Work out the finished part from the listing and answer in its coordinate system (mm). A direction names the side the tool comes from. Give positions to 0.01 mm unless a question says otherwise; leave off trailing zeros. Loops run counter-clockwise (first coordinate to the right, second up) from the corner with the lowest first, then second, coordinate; pieces in that order, holes last. Notation, with made-up numbers: M -36.75,63 L 13.25,63 A28 ccw 13.25,89 Z; hole C 53,-11 d11. An arc over 180 degrees is marked long. Write item = value, one per line. Start each with the question number.
1. Section B-B on x = 0 is taken. Determine the outline of the cut face in (y, z) (1 decimal).
2. Section D-D on y = -59 is taken. Determine the outline of the cut face in (x, z) (3 decimals).
3. Section C-C on y = -7 is taken. Determine the outline of the cut face in (x, z).
4. Flat-ended cylindrical pins translate along their axes: pin 1 Ø12 at (x, z) = (21, 14.5) entering from -Y; pin 2 Ø4 at (y, z) = (-84, 22) entering from +X; pin 3 Ø2 at (x, z) = (11, -22.5) entering from -Y; pin 4 Ø6 at (y, z) = (-78.5, 31) entering from -X. Find the tip coordinate at first contact, or state that the pin passes through.
5. For faces 4 (the face through (-7.989, -88.726, 25.368)), 5 (the face through (-10, -76.2, -27)), 6 (the face through (-5.68, -12.52, -25.57)), 7 (the face through (-25.3, 0, 4)), determine the directions among +Z, -Z, +X, -X, +Y, -Y from which every point of the face is accessible in a straight line to the end or side of a thin tool.
6. The mould has two halves that part along Y. Classify faces 1 (the face through (27.5, -89.08, -6.11)), 2 (the face through (20, -76.2, -16)), 3 (the face through (-8.948, -50.444, -40.293)): released by +Y, released by -Y, zero draft, split by the parting line, or undercut.
7. Section A-A on z = 0 is taken. Determine the outline of the cut face in (x, y) (1 decimal).
8. Consider L1, parallel to Z at x = 0, y = -11.5; L2, parallel to Y at x = -37, z = -13.5; L3, parallel to Z at x = 0, y = -63 (3 decimals). Determine where each line is inside the solid, lowest interval first. Write a range as [from, to].
```python
from build123d import *

# Parameters (mm, degrees)
F0_R      = 26.19375
F0_R_2    = 25.4
F1_DEPTH  = 25.4
F2_R      = 41.275
F3_DEPTH  = 50.8
F3_FACE_R = 25.4
F6_DEPTH  = 76.2


with BuildPart() as f1:
    # F0 (on Front) → F1 (new body)
    with BuildSketch(Plane.XZ):
        Circle(F0_R)
        Circle(F0_R_2, mode=Mode.SUBTRACT)
    extrude(amount=F1_DEPTH)

    # F2 (on face) → F3 (join)
    with BuildSketch(Plane.XZ.offset(25.4)):
        Circle(F2_R)
    extrude(amount=F3_DEPTH)

    # F4 (on Right) → F5 (revolve)
    with BuildSketch(Plane.YZ):
        Polygon((-76.2, 28.575), (-101.6, 27.78125), (-101.606704, 26.19375), (-76.2, 26.9875), align=None)
    revolve(axis=Axis((0, -38.1, 0), (0, -1, 0)))

    # F3_face (on face) → F6 (cut)
    with BuildSketch(Plane(origin=(0, -25.4, 0), x_dir=(1, 0, 0), z_dir=(0, 1, 0))):
        Circle(F3_FACE_R)
    extrude(amount=-F6_DEPTH, mode=Mode.SUBTRACT)


solid = f1.part
```
Verdict:
q1.outline = M -101.6,-27.8 L -76.2,-28.6 L -76.2,-41.3 L -25.4,-41.3 L -25.4,-26.2 L 0,-26.2 L 0,-25.4 L -76.2,-25.4 L -76.2,-27 L -101.6,-26.2 Z; M -101.6,26.2 L -76.2,27 L -76.2,25.4 L 0,25.4 L 0,26.2 L -25.4,26.2 L -25.4,41.3 L -76.2,41.3 L -76.2,28.6 L -101.6,27.8 Z
q2.outline = C 0,0 d82.55; hole C 0,0 d50.8
q3.outline = C 0,0 d52.39; hole C 0,0 d50.8
q4.pin_1 = -101.61
q4.pin_2 = 20.07
q4.pin_3 = -76.2
q4.pin_4 = -29.3
q5.face_4 = none
q5.face_5 = -Y
q5.face_6 = +Y
q5.face_7 = +Z, -Z, +X, -X, +Y
q6.face_1 = released by -Y
q6.face_2 = undercut
q6.face_3 = zero draft
q7.outline = M -41.3,-76.2 L -28.6,-76.2 L -27.8,-101.6 L -26.2,-101.6 L -27,-76.2 L -25.4,-76.2 L -25.4,0 L -26.2,0 L -26.2,-25.4 L -41.3,-25.4 Z; M 25.4,-76.2 L 27,-76.2 L 26.2,-101.6 L 27.8,-101.6 L 28.6,-76.2 L 41.3,-76.2 L 41.3,-25.4 L 26.2,-25.4 L 26.2,0 L 25.4,0 Z
q8.L1 = [-26.19, -25.4], [25.4, 26.19]
q8.L2 = [-76.2, -25.4]
q8.L3 = [-41.275, -25.4], [25.4, 41.275]
